Check sheet for the modelled part. Datum: model origin and axes. Units: mm. A direction names the side the tool comes from. Coordinates: 2 decimals unless noted, no trailing zeros. Loops run counter-clockwise (first coordinate to the right, second up) from the corner with the lowest first, then second, coordinate; pieces in that order, holes last. Notation, with made-up numbers: (87, -31) -> (142, -31) arc R22 cw to (142, 2) -> close; hole circle Ø10 at (70, 54.25). An arc over 180 degrees is marked (long way). Use CSV: the item, a comma, the result in double quotes. Start each with the question number.
1. Sectioned sample at D-D, the plane z = -76. Record the cut outline in (x, y).
2. Release check for a two-part mould opening along X. For faces 3 (the face through (7.961, -35.853, -3.71)), 4 (the face through (0, 0, -49.53)), 5 (the face through (0, 0, -164.592)), 6 (the face through (3.13, 23.82, 2.55)) record: pulls with the +X half, pulls with the -X half, needs draft (parallel to the pull), parting line crosses it, or undercut.
3. Sectioned sample at A-A, the plane y = 0. Record the cut outline in (x, z).
4. Set-up check for faces 1 (the face through (-8, -24, 53.194)), 2 (the face through (-8, -24, -62.23)): record each of +Z, -Z, +X, -X, +Y, -Y from which the full face is reachable in a straight line by a thin tool's end or side.
5. Sectioned sample at C-C, the plane z = 9.5. Record the cut outline in (x, y), and give its area (3 significant figures).
6. Thickness scan on L1, parallel to Y at x = 0, z = -4; L2, parallel to Z at x = -27, y = 11; L3, parallel to Z at x = 5.5, y = -5.5. Record the ranges inside material, lowest first.
7. Gauge pin test, flat ends, axial feed: pin 1 (5 mm diameter, centred on y = 7.5, z = -22, fed in from +X); pin 2 (1 mm diameter, centred on x = -10, z = -7, fed in from +Y); pin 3 (4 mm diameter, centred on x = 24, z = 0, fed in from +Y). Record the tip position at first contact, or that the pin passes through.
8. Sectioned sample at B-B, the plane x = -15. Record the cut outline in (y, z), and give its area (3 significant figures).
```python
from build123d import *

# Parameters (mm, degrees)
F0_W     = 36.7259010673
F0_H     = 115.4242623597
F2_T     = -12.7
F3_DEPTH = 115.062


with BuildPart() as f1:
    # F0 (on Front) → F1 (revolve)
    with BuildSketch(Plane.XZ):
        with Locations((-18.3629505336, -4.5178690925)):
            Rectangle(F0_W, F0_H)
    revolve(axis=Axis((0, 0, -4.5178690925), (0, 0, -1)))

    # F2
    f2_openings = [f1.faces().sort_by_distance(p)[0] for p in [
        (0, 0, 53.194262),
    ]]
    offset(amount=F2_T, openings=f2_openings)

    # F3 (add): a face of the model
    f3_faces = [f1.faces().sort_by_distance(p)[0] for p in [
        (0, 0, -49.5300002724),
    ]]
    extrude(f3_faces, amount=-F3_DEPTH)


solid = f1.part
```
Completed:
1,outline,"circle Ø48.05 at (0, 0)"
2,face 3,"parting line crosses it"
2,face 4,"undercut"
2,face 5,"needs draft"
2,face 6,"undercut"
3,outline,"(-36.73, -62.23) -> (-24.03, -62.23) -> (-24.03, -164.59) -> (24.03, -164.59) -> (24.03, -62.23) -> (36.73, -62.23) -> (36.73, 53.19) -> (24.03, 53.19) -> (24.03, -49.53) -> (-24.03, -49.53) -> (-24.03, 53.19) -> (-36.73, 53.19) -> close"
4,face 1,"+Z, +X, -X, +Y, -Y"
4,face 2,"-Z"
5,outline,"circle Ø73.45 at (0, 0); hole circle Ø48.05 at (0, 0)"
5,area,"2,420 mm²"
6,L1,"-36.73 to -24.03, 24.03 to 36.73"
6,L2,"-62.23 to 53.19"
6,L3,"-164.59 to -49.53"
7,pin 1,"x = 36.38"
7,pin 2,"y = 35.48"
7,pin 3,"y = 29.41"
8,outline,"(-33.52, -62.23) -> (-18.77, -62.23) -> (-18.77, -164.59) -> (18.77, -164.59) -> (18.77, -62.23) -> (33.52, -62.23) -> (33.52, 53.19) -> (18.77, 53.19) -> (18.77, -49.53) -> (-18.77, -49.53) -> (-18.77, 53.19) -> (-33.52, 53.19) -> close"
8,area,"7,730 mm²"
